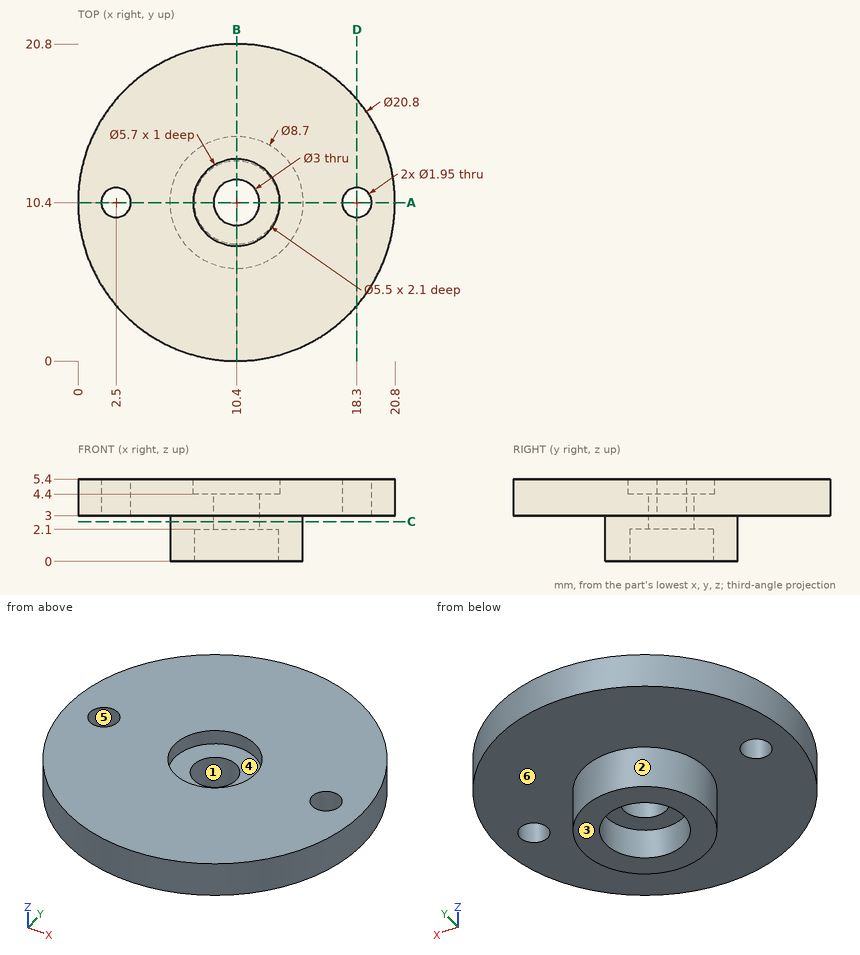
Design review of the part shown in the three views and the two pictorial views. Dimensions are in mm from the part's minimum x, y and z. A direction names the side the tool comes from. Give positions to 0.01 mm unless a question says otherwise; leave off trailing zeros. Write each loop counter-clockwise with the first axis right and the second up, starting at its lowest first coordinate (ties: lowest second). Pieces come first, ordered by that corner, then holes.
Item 1: Take a section at C-C (z = 2.6). Give the boundary of the cut face in (x, y).
Item 2: Machinability: for the marked faces 4, 5 and 6, which of the approach directions +Z, -Z, +X, -X, +Y, -Y give a long, thin tool a straight path to every point of the face, cutting with its end or side? Answer none if there is none.
Item 3: Wall thickness on probe 1 along Y at (x, z) = (10.4, 1.45); probe 2 along Y at (x, z) = (10.4, 5.2); probe 3 along Z at (x, y) = (18.25, 15.75): over which ranges is each line inside the solid? List them lowest first.
Item 4: Insertion check: P1, Ø3, axis at x = 11.5, y = 10.5, coming from the +Z side; P2, Ø1.8, axis at x = 10.4, y = 10.4, coming from the +Z side; P3, Ø1.5, axis at y = 14.5, z = 1.5, coming from the +X side; P4, Ø5, axis at x = 10.4, y = 10.4, coming from the -Z side. Each pin has a flat end and moves straight along its axis. Give the tip position at first contact, or say it passes through.
Item 5: The part is to be moulded in two halves that separate along Y. For the marked faces 1, 2 and 3, say which applies: +Y half, -Y half, draft (parallel to the pull), parting line (faces both ways), or undercut.
Item 6: Take a section at B-B (x = 10.4). Give the boundary of the cut face in (y, z), and give its area (3 significant figures).
Item 7: Take a section at D-D (x = 18.3). Give the boundary of the cut face in (y, z) (3 decimals).
Item 8: Take a section at A-A (y = 10.4). Give the boundary of the cut face in (x, z) (3 decimals).
Established:
1. outline: circle Ø8.7 at (10.4, 10.4); hole circle Ø3 at (10.4, 10.4)
2. face 4: +Z
2. face 5: +Z, -Z
2. face 6: -Z
3. probe 1: y = 6.05 to 7.65, 13.15 to 14.75
3. probe 2: y = 0 to 7.55, 13.25 to 20.8
3. probe 3: z = 3 to 5.4
4. P1: stops at z = 4.4
4. P2: passes through
4. P3: stops at x = 13.17
4. P4: stops at z = 2.1
5. face 1: undercut
5. face 2: parting line
5. face 3: draft
6. outline: (0, 3) - (6.05, 3) - (6.05, 0) - (7.65, 0) - (7.65, 2.1) - (8.9, 2.1) - (8.9, 4.4) - (7.55, 4.4) - (7.55, 5.4) - (0, 5.4) - close; (11.9, 2.1) - (13.15, 2.1) - (13.15, 0) - (14.75, 0) - (14.75, 3) - (20.8, 3) - (20.8, 5.4) - (13.25, 5.4) - (13.25, 4.4) - (11.9, 4.4) - close
6. area: 51.9 mm2
7. outline: (3.636, 3) - (9.425, 3) - (9.425, 5.4) - (3.636, 5.4) - close; (11.375, 3) - (17.164, 3) - (17.164, 5.4) - (11.375, 5.4) - close
8. outline: (0, 3) - (1.525, 3) - (1.525, 5.4) - (0, 5.4) - close; (3.475, 3) - (6.05, 3) - (6.05, 0) - (7.65, 0) - (7.65, 2.1) - (8.9, 2.1) - (8.9, 4.4) - (7.55, 4.4) - (7.55, 5.4) - (3.475, 5.4) - close; (11.9, 2.1) - (13.15, 2.1) - (13.15, 0) - (14.75, 0) - (14.75, 3) - (17.325, 3) - (17.325, 5.4) - (13.25, 5.4) - (13.25, 4.4) - (11.9, 4.4) - close; (19.275, 3) - (20.8, 3) - (20.8, 5.4) - (19.275, 5.4) - close
